Read the model definition and answer for the solid it produces. Units are mm, in the model's axes. A direction names the side the tool comes from. Round coordinates to 2 decimals unless told otherwise and drop trailing zeros. Order: outer loops, then holes, each group sorted by start corner. A loop starts at its lowest first (then second) coordinate and runs counter-clockwise, first axis right, second up. Notation, with made-up numbers: (55, 3) -> (84, 3) arc R18 cw to (84, 22) -> close; hole circle Ø9 at (-5, -39). An arc over 180 degrees is marked (long way). One line per item, written item: value. Start each with the question number.
1. Section D-D (y = 16) is taken. Give the vertices of the cut face in (x, z).
2. Section C-C (z = 2.4) is taken. Give the vertices of the cut face in (x, y), then the cut area to 3 significant figures.
3. Section A-A (x = -15) is taken. Give the vertices of the cut face in (y, z).
4. The mould has two halves that part along Y. Classify faces 1 (the face through (0, 0, 3)), 2 (the face through (-22.5, -24, 1.5)), 3 (the face through (15, -17.6, 1.5)): released by +Y, released by -Y, zero draft, split by the parting line, or undercut.
5. For faces 4 (the face through (17.1, 0, 1)), 5 (the face through (-25, 2, 1)), determine the directions among +Z, -Z, +X, -X, +Y, -Y from which every point of the face is accessible in a straight line to the end or side of a thin tool.
6. Consider line 1 (X direction, y = -12, z = 2.15); line 2 (Y direction, x = 15, z = 2); line 3 (X direction, y = -17, z = 0.55). Determine where each line is inside the solid, lowest interval first.
7. Section B-B (y = -10.5) is taken. Give the vertices of the cut face in (x, z), then the cut area to 3 significant figures.
from build123d import *

# Parameters (mm, degrees)
RESSALTO_EXTRUS_O1_DEPTH = 3


with BuildPart() as part:
    # Esboço1 → Ressalto-extrusão1 (new body)
    with BuildSketch(Plane.XY):
        Polygon((-25, -21.5), (-25, 26.5), (25, 26.5), (25, -21.5), (20, -26.5), (-20, -26.5), align=None)
        with BuildLine():
            Line((17.1, 14.5), (17.1, -15.5))
            ThreePointArc((17.1, -15.5), (15, -17.6), (12.9, -15.5))
            Line((12.9, -15.5), (12.9, 14.5))
            ThreePointArc((12.9, 14.5), (15, 16.6), (17.1, 14.5))
        make_face(mode=Mode.SUBTRACT)
        with BuildLine():
            Line((-17.1, 14.5), (-17.1, -15.5))
            ThreePointArc((-17.1, -15.5), (-15, -17.6), (-12.9, -15.5))
            Line((-12.9, -15.5), (-12.9, 14.5))
            ThreePointArc((-12.9, 14.5), (-15, 16.6), (-17.1, 14.5))
        make_face(mode=Mode.SUBTRACT)
    extrude(amount=RESSALTO_EXTRUS_O1_DEPTH)


solid = part.part
Answer:
1. outline: (-25, 0) -> (-16.47, 0) -> (-16.47, 3) -> (-25, 3) -> close; (-13.53, 0) -> (13.53, 0) -> (13.53, 3) -> (-13.53, 3) -> close; (16.47, 0) -> (25, 0) -> (25, 3) -> (16.47, 3) -> close
2. outline: (-25, -21.5) -> (-20, -26.5) -> (20, -26.5) -> (25, -21.5) -> (25, 26.5) -> (-25, 26.5) -> close; hole (-17.1, -15.5) arc R2.1 ccw to (-12.9, -15.5) -> (-12.9, 14.5) arc R2.1 ccw to (-17.1, 14.5) -> close; hole (12.9, -15.5) arc R2.1 ccw to (17.1, -15.5) -> (17.1, 14.5) arc R2.1 ccw to (12.9, 14.5) -> close
2. area: 2,350 mm^2
3. outline: (-26.5, 0) -> (-17.6, 0) -> (-17.6, 3) -> (-26.5, 3) -> close; (16.6, 0) -> (26.5, 0) -> (26.5, 3) -> (16.6, 3) -> close
4. face 1: zero draft
4. face 2: released by -Y
4. face 3: undercut
5. face 4: +Z, -Z
5. face 5: +Z, -Z, -X, +Y, -Y
6. line 1: -25 to -17.1, -12.9 to 12.9, 17.1 to 25
6. line 2: -26.5 to -17.6, 16.6 to 26.5
6. line 3: -25 to -16.47, -13.53 to 13.53, 16.47 to 25
7. outline: (-25, 0) -> (-17.1, 0) -> (-17.1, 3) -> (-25, 3) -> close; (-12.9, 0) -> (12.9, 0) -> (12.9, 3) -> (-12.9, 3) -> close; (17.1, 0) -> (25, 0) -> (25, 3) -> (17.1, 3) -> close
7. area: 125 mm^2
